The model under review builds one solid part; all positions refer to its coordinate system, in mm. Give positions to 0.01 mm unless a question says otherwise; leave off trailing zeros. Loops run counter-clockwise (first coordinate to the right, second up) from the corner with the lowest first, then second, coordinate; pieces in that order, holes last. Notation, with made-up numbers: (-8, 45.25) - (1, 45.25) arc R16 ccw to (1, 56.25) - close; hole circle Ø3 at (-22.5, -16.75). An arc over 180 degrees is marked (long way). Return JSON: item names as keys, results as strings. Group by question number.
Autodesk Inventor part; units mm, degrees
ref_plane "YZ Plane" through (0, 0, 0) normal (1, 0, 0) x (0, 1, 0)
ref_plane "XZ Plane" through (0, 0, 0) normal (0, 1, 0) x (-1, 0, 0)
ref_plane "XY Plane" through (0, 0, 0) normal (0, 0, 1) x (1, 0, 0)
sketch "スケッチ1" plane through (0, 0, 0) normal (0, 0, 1) x (1, 0, 0)
  arc A0 (-2.6047, -14.7721) -> (15, 0) centre (0, 0) ccw construction
  arc A1 (-2.0751, -11.7685) -> (11.5542, -3.05) centre (0, 0) ccw
  arc A2 (-2.0751, -11.7685) -> (-2.602, -11.7221) centre (-2.6047, -14.7721) ccw
  line L0 (0, 0) -> (-6, 0) construction
  line L1 (0, 3.05) -> (-6, 3.05)
  line L2 (-6, -3.05) -> (0, -3.05)
  arc A3 (0, -3.05) -> (0, 3.05) centre (0, 0) ccw
  arc A4 (-6, 3.05) -> (-6, -3.05) centre (-6, 0) ccw
  line L3 (15, 0) -> (9, 0) construction
  line L4 (15, 3.05) -> (9, 3.05)
  arc A5 (9, 3.05) -> (9, -3.05) centre (9, 0) ccw
  line L5 (-169.2784, 7.05) -> (0.7216, 7.05)
  line L6 (-169.2784, 7.05) -> (-151.6413, -2.95)
  line L7 (-2.602, -11.7221) -> (-151.6413, -2.95)
  arc A6 (17.9444, -0.7957) -> (15, 3.05) centre (15, 0) ccw
  line L8 (9, -3.05) -> (11.5542, -3.05)
  line L9 (14.6866, -3.05) -> (14.3582, -3.05)
  circle A7 centre (21.3232, -1.7088) radius 1.25
  arc A8 (17.9444, -0.7957) -> (23.4882, 1.0412) centre (21.3232, -1.7088) ccw
  line L10 (0.7216, 7.05) -> (15.8557, 7.05)
  line L11 (15.8557, 7.05) -> (23.4882, 1.0412)
  point P0 (-3, 0)
  point P1 (12, 0)
  dimension "d0" = 15
  dimension "d1" = 6.1
  dimension "d2" = 6
  dimension "d3" = 6.1
  dimension "d4" = 6
  dimension "d5" = 6.1
  dimension "d6" = 100
  dimension "d8" = 4
  dimension "d9" = 10
  dimension "d17" = 2.5
  dimension "d20" = 170
extrude "押し出し1" add sketch "スケッチ1" along normal blind 5
fillet "フィレット1" radius 2 2 edges at (-169.2784, 7.05, 2.5) (-151.6413, -2.95, 2.5)
fillet "フィレット3" radius 1 1 edges at (11.5542, -3.05, 2.5)
properties part number "新型４ウイング" material "ポリカーボネート、クリア"
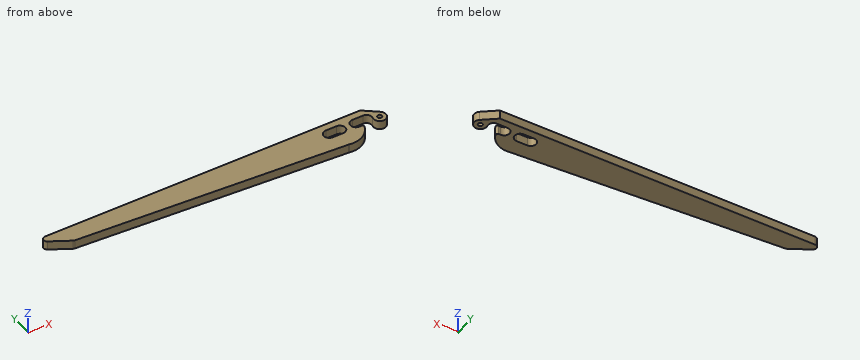
1) For pin 1 Ø2.5 at (x, z) = (13.5, 3.5) entering from -Y; pin 2 Ø1.5 at (y, z) = (4.5, 2) entering from +X, all flat-tipped, find the tip position at first contact; note any pin that passes through.
2) We need section A-A, the plane z = 1.3. Write out the cut boundary in (x, y).
3) To check wall thickness, follow line 1 (X direction, y = 2.5, z = 1.2); line 2 (X direction, y = -0.75, z = 1.15); line 3 (X direction, y = 0, z = 3.5). State the ranges of each line that lie inside material, in increasing order.
4) We need section B-B, the plane x = -119. Write out the cut boundary in (y, z).
5) We need section C-C, the plane y = -9.5. Write out the cut boundary in (x, z).
Findings:
{
 "1": {"pin 1": "stops at y = 3.05", "pin 2": "stops at x = 20.05"},
 "2": {"outline": "(-162.68, 3.31) - (-152.05, -2.72) arc R2 ccw to (-151.18, -2.98) - (-2.6, -11.72) arc R3.06 cw to (-2.08, -11.77) arc R11.95 ccw to (11.1, -4.42) arc R1 ccw to (10.17, -3.05) - (9, -3.05) arc R3.05 cw to (9, 3.05) - (15, 3.05) arc R3.05 cw to (17.94, -0.8) arc R3.5 ccw (long way) to (23.49, 1.04) - (15.86, 7.05) - (-161.7, 7.05) arc R2 ccw to start; hole (-6, -3.05) - (0, -3.05) arc R3.05 ccw to (0, 3.05) - (-6, 3.05) arc R3.05 ccw to start; hole circle Ø2.5 at (21.32, -1.71)"},
 "3": {"line 1": "x = -161.25 to -7.75, 1.75 to 7.25, 16.75 to 21.64", "line 2": "x = -155.52 to -8.96, 2.96 to 6.04, 17.96 to 20.52, 22.13 to 24.69", "line 3": "x = -156.84 to -9.05, 3.05 to 5.95, 18.05 to 24.38"},
 "4": {"outline": "(-4.87, 0) - (7.05, 0) - (7.05, 5) - (-4.87, 5) - close"},
 "5": {"outline": "(-40.36, 0) - (7.25, 0) - (7.25, 5) - (-40.36, 5) - close"}
}
